from build123d import *

# Parameters (mm, degrees)
F1_DEPTH = 54
F3_DEPTH = 16
F4_R     = 8
F5_DEPTH = 22
F7_DEPTH = 42.001


with BuildPart() as f1:
    # F0 (on Front) → F1 (new body)
    with BuildSketch(Plane.XZ):
        Polygon((0, 6), (0, 0), (24, 0), (24, 6), (34, 6), (34, 16), (110, 16), (110, 32.019238), (65, 58), (-10, 58), (-10, 6), align=None)
    extrude(amount=F1_DEPTH)

    # F2 (on face) → F3 (cut)
    with BuildSketch(Plane.XZ.offset(54)):
        Polygon((65, 58), (-10, 58), (-10, 46), (34, 46), (34, 16), (110, 16), (110, 32.019238), align=None)
    extrude(amount=-F3_DEPTH, mode=Mode.SUBTRACT)

    # F4 (on face) → F5 (cut)
    with BuildSketch(Plane.XZ.offset(54)):
        with Locations((12, 28)):
            Circle(F4_R)
    extrude(amount=-F5_DEPTH, mode=Mode.SUBTRACT)

    # F6 (on face) → F7 (cut, through all)
    with BuildSketch(Plane(origin=(0, 0, 16), x_dir=(1, 0, 0), z_dir=(0, 0, -1))):
        Polygon((110, 20), (80, 0), (110, 0), align=None)
    extrude(amount=-F7_DEPTH, mode=Mode.SUBTRACT)


solid = f1.part
The model under review builds one solid part; all positions refer to its coordinate system, in mm. A direction names the side the tool comes from. Coordinates: 2 decimals unless noted, no trailing zeros. Loops run counter-clockwise (first coordinate to the right, second up) from the corner with the lowest first, then second, coordinate; pieces in that order, holes last.
(1) Insertion check: P1, Ø17.5, axis at x = 5.5, y = -50, coming from the +Z side; P2, Ø21, axis at x = 49, z = 30.5, coming from the -Y side; P3, Ø4, axis at y = -46, z = 45, coming from the +X side. Each pin has a flat end and moves straight along its axis. Give the tip position at first contact, or say it passes through.
Determined:
P1: stops at z = 46
P2: stops at y = -38
P3: stops at x = 34
(2) Wall thickness on L1, parallel to Z at x = 12, y = -41; L2, parallel to X at y = -14, z = 13.5; L3, parallel to Z at x = 12, y = -37: over which ranges is each line inside the solid? List them lowest first.
Determined:
L1: z = 0 to 20, 36 to 46
L2: x = -10 to 34
L3: z = 0 to 20, 36 to 58
(3) Consider section C-C, the plane x = 12. Give the boundary of the cut face in (y, z), plus the area to 3 significant figures.
Determined:
outline: (-54, 0) - (0, 0) - (0, 58) - (-38, 58) - (-38, 46) - (-54, 46) - (-54, 36) - (-32, 36) - (-32, 20) - (-54, 20) - close
area: 2,590 mm2
(4) Tool access review of faces 1 (the flat face through (24, -27, 3)), 2 (the flat face through (12, -32, 28)), 3 (the flat face through (0, -27, 3)), 4 (the flat face through (110, -29, 24)): name each direction out of +Z, -Z, +X, -X, +Y, -Y from which nothing blocks a thin tool from reaching the whole face with its end or side.
Determined:
face 1: -Z, +X, +Y, -Y
face 2: -Y
face 3: -Z, -X, +Y, -Y
face 4: +Z, -Z, +X, +Y, -Y
(5) Consider section D-D, the plane y = -28. Give the boundary of the cut face in (x, z).
Determined:
outline: (-10, 6) - (0, 6) - (0, 0) - (24, 0) - (24, 6) - (34, 6) - (34, 16) - (110, 16) - (110, 32.02) - (65, 58) - (-10, 58) - close
(6) Consider section A-A, the plane y = -40.5. Give the boundary of the cut face in (x, z), plus the area to 3 significant figures.
Determined:
outline: (-10, 6) - (0, 6) - (0, 0) - (24, 0) - (24, 6) - (34, 6) - (34, 46) - (-10, 46) - close; hole circle Ø16 at (12, 28)
area: 1,700 mm2
(7) Draft analysis for pull direction Z (two halves, no side actions). For faces 5 (the flat face through (34, 0, 36)), 6 (the cylindrical face through (10.959, -43.154, 35.932)), 7 (the flat face through (-5, -27, 6)), 8 (the flat face through (12, -46, 46)), state which applies: +Z half, -Z half, draft (parallel to the pull), parting line (faces both ways), or undercut.
Determined:
face 5: draft
face 6: undercut
face 7: -Z half
face 8: +Z half
(8) Consider section B-B, the plane z = 28. Give the boundary of the cut face in (x, y), plus the area to 3 significant figures.
Determined:
outline: (-10, -54) - (4, -54) - (4, -32) - (20, -32) - (20, -54) - (34, -54) - (34, -38) - (110, -38) - (110, -20) - (80, 0) - (-10, 0) - close
area: 4,610 mm2
